Autodesk Inventor part; units mm, degrees
ref_plane "YZ Plane" through (0, 0, 0) normal (1, 0, 0) x (0, 1, 0)
ref_plane "XZ Plane" through (0, 0, 0) normal (0, 1, 0) x (-1, 0, 0)
ref_plane "XY Plane" through (0, 0, 0) normal (0, 0, 1) x (1, 0, 0)
sketch "Sketch1" plane through (0, 0, 0) normal (0, 0, 1) x (1, 0, 0)
  line L0 (0, 0) -> (0, 15.875)
  line L1 (0, 15.875) -> (0.7937, 15.875)
  line L2 (0.7937, 15.875) -> (0.7938, 0.7937)
  line L3 (0.7938, 0.7937) -> (15.875, 0.7937)
  line L4 (15.875, 0.7937) -> (15.875, 0)
  line L5 (15.875, 0) -> (0, 0)
  dimension "d0" = 15.875
  dimension "d1" = 0.7937
extrude "Extrusion1" add sketch "Sketch1" along normal blind 228.6
sketch "Sketch2" plane through (0.7938, 0.7937, 0) normal (0, 1, 0) x (1, 0, 0)
  line L0 (0, 0) -> (15.0812, 0)
  line L1 (15.0812, -228.6) -> (0, -228.6)
  line L2 (7.5406, 0) -> (7.5406, -228.6) construction
  circle A0 centre (7.5406, -9.525) radius 1.5875
  circle A1 centre (7.5406, -79.375) radius 1.5875
  circle A2 centre (7.5406, -149.225) radius 1.5875
  circle A3 centre (7.5406, -219.075) radius 1.5875
  point P0 (-0.7938, 0)
  dimension "d4" = 9.525
  dimension "d5" = 3.175
  dimension "d6" = 228.6
  dimension "d9" = 69.85
sketch "Sketch3" plane through (0.7938, 0.7937, 0) normal (1, 0, 0) x (0, 0, -1)
  line L0 (0, 15.0812) -> (0, 0)
  line L1 (-228.6, 0) -> (-228.6, 15.0812)
  line L2 (-228.6, 7.5406) -> (0, 7.5406) construction
  circle A0 centre (-9.525, 7.5406) radius 1.5875
  circle A1 centre (-79.375, 7.5406) radius 1.5875
  circle A2 centre (-149.225, 7.5406) radius 1.5875
  circle A3 centre (-219.075, 7.5406) radius 1.5875
  point P0 (0, -0.7937)
  dimension "d14" = 3.175
  dimension "d15" = 9.525
  dimension "d16" = 228.6
  dimension "d19" = 69.85
extrude "Extrusion2" cut sketch "Sketch2" against normal through all
extrude "Extrusion3" cut sketch "Sketch3" against normal through all
properties part number "Hopper Bracing Front Bottom P6" material "Aluminum 6061"
Geometry check sheet. Reference: the model listing, model coordinates, mm. A direction names the side the tool comes from. Round coordinates to 2 decimals unless told otherwise and drop trailing zeros. Order: outer loops, then holes, each group sorted by start corner. A loop starts at its lowest first (then second) coordinate and runs counter-clockwise, first axis right, second up. Notation, with made-up numbers: (30, 10) -> (78, 10) arc R25 cw to (78, 36) -> close; hole circle Ø9 at (74, -19). An arc over 180 degrees is marked (long way). Return JSON: item names as keys, results as strings. Group by question number.
Q1. Section check A-A, the plane z = 180. Record the boundary of the cut face in (x, y) (3 decimals), plus the area to 3 significant figures.
Q2. Section check B-B, the plane x = 13.5. Record the boundary of the cut face in (y, z).
Q3. Material ranges on probe 1 along X at (y, z) = (7.5, 215), recorded low to high. Write a range as from..to.
Q4. Tool access check on faces 1 (the flat face through (4.4, 0.3, 228.6)), 2 (the flat face through (8, 0.794, 113)). Record the directions out of +Z, -Z, +X, -X, +Y, -Y that give a thin tool (end or side, any length) a straight path to the whole face; none if there is none.
Q5. Gauge pin test, flat ends, axial feed: pin 1 (8 mm diameter, centred on y = 11.5, z = 183, fed in from -X); pin 2 (3.5 mm diameter, centred on x = 8.33, z = 9.52, fed in from +Y); pin 3 (4 mm diameter, centred on y = 11.5, z = 102, fed in from +X). Record the tip position at first contact, or that the pin passes through.
Numbers:
{
 "1": {"outline": "(0, 0) -> (15.875, 0) -> (15.875, 0.794) -> (0.794, 0.794) -> (0.794, 15.875) -> (0, 15.875) -> close", "area": "24.6 mm^2"},
 "2": {"outline": "(0, 0) -> (0.79, 0) -> (0.79, 228.6) -> (0, 228.6) -> close"},
 "3": {"probe 1": "0..0.79"},
 "4": {"face 1": "+Z, +X, -X, +Y, -Y", "face 2": "+Z, -Z, +X, +Y"},
 "5": {"pin 1": "x = 0", "pin 2": "y = 0.79", "pin 3": "x = 0.79"}
}
